Check sheet for the modelled part. Datum: model origin and axes. Units: mm. A direction names the side the tool comes from. Give positions to 0.01 mm unless a question says otherwise; leave off trailing zeros. Order: outer loops, then holes, each group sorted by start corner. A loop starts at its lowest first (then second) coordinate and runs counter-clockwise, first axis right, second up. Notation, with made-up numbers: (0, 64) - (29, 64) arc R16 ccw to (29, 79) - close; hole circle Ø11 at (25.5, 80.5). An arc over 180 degrees is marked (long way). Answer in a Markdown table with one row per item.
from build123d import *

# Parameters (mm, degrees)
BASE_DEPTH              = 0.8636
TIER1_DEPTH             = 0.3556
CHAMFER1_SIZE           = 0.3556
SKETCH3_R               = 1
BUTTON_DEPTH            = 0.3048
BUTTONC_R               = 0.0508
SKETCH4_W               = 5.08
SKETCH4_H               = 1.524
BOTTOM_CUT_DEPTH        = 0.0508
PINS_START              = -0.4445
SKETCH6_W               = 0.508
SKETCH6_H               = 0.1524
PINS_DEPTH              = 0.508
MIRROR2_START           = -0.4445
MIRROR2_COPY_1_SKETCH_W = 0.508
MIRROR2_COPY_1_SKETCH_H = 0.1524
MIRROR2_COPY_1_DEPTH    = 0.508


with BuildPart() as part:
    # Sketch1 → Base (new body)
    with BuildSketch(Plane.XY):
        Polygon((-1.3462, 2.54), (1.3462, 2.54), (2.54, 1.3462), (2.54, -1.3462), (1.3462, -2.54), (-1.3462, -2.54), (-2.54, -1.3462), (-2.54, 1.3462), align=None)
    extrude(amount=BASE_DEPTH)

    # Sketch2 → Tier1 (add)
    with BuildSketch(Plane.XY.offset(0.8636)):
        Polygon((-1.093695412, 1.9304), (-1.9304, 1.093695412), (-1.9304, -1.093695412), (-1.093695412, -1.9304), (1.093695412, -1.9304), (1.9304, -1.093695412), (1.9304, 1.093695412), (1.093695412, 1.9304), align=None)
    extrude(amount=TIER1_DEPTH)

    # Chamfer1
    chamfer1_edges = [part.edges().sort_by_distance(p)[0] for p in [
        (-1.512047706, 1.512047706, 1.2192),
        (0, 1.9304, 1.2192),
        (1.512047706, 1.512047706, 1.2192),
        (1.9304, 0, 1.2192),
        (1.512047706, -1.512047706, 1.2192),
        (0, -1.9304, 1.2192),
        (-1.512047706, -1.512047706, 1.2192),
        (-1.9304, 0, 1.2192),
    ]]
    chamfer(chamfer1_edges, length=CHAMFER1_SIZE - 0.0001)  # a hair under: the kernel refuses the full size

    # Sketch3 → Button (add)
    with BuildSketch(Plane.XY.offset(1.2192)):
        Circle(SKETCH3_R)
    extrude(amount=BUTTON_DEPTH)

    # ButtonC
    buttonc_edges = [part.edges().sort_by_distance(p)[0] for p in [
        (-1, 0, 1.524),
    ]]
    fillet(buttonc_edges, radius=BUTTONC_R)

    # Sketch4 → Bottom cut (cut)
    with BuildSketch(Plane(origin=(0, 0, 0), x_dir=(-1, 0, 0), z_dir=(0, 0, -1))):
        Rectangle(SKETCH4_W, SKETCH4_H)
    extrude(amount=-BOTTOM_CUT_DEPTH, mode=Mode.SUBTRACT)

    # Sketch6 → pins (add)
    with BuildSketch(Plane.XZ.offset(2.54).offset(PINS_START)):
        with Locations((-1.0922, 0.3048)):
            Rectangle(SKETCH6_W, SKETCH6_H)
        Polygon((-1.3462, 0.2286), (-1.3462, 0.381), (-2.2352, 0.381), (-2.2352, 0.3048), (-2.2352, 0.2286), align=None)
        with BuildLine():
            Line((-2.2352, 0.3048), (-2.2352, 0.381))
            add(Edge.make_bspline(
                [(-2.2352, 0.381), (-2.307735088, 0.381), (-2.477008689, 0.347316172), (-2.556176281, 0.222815828), (-2.591192004, 0.183226461), (-2.642048799, 0.15910292), (-2.712296659, 0.1524), (-2.742, 0.1524)],
                knots=[0, 0, 0, 0, 0.25, 0.5, 0.75, 0.875, 1, 1, 1, 1], degree=3))
            Line((-2.742, 0.1524), (-2.742, 0.0762))
            add(Edge.make_bspline(
                [(-2.2352, 0.3048), (-2.573866667, 0.3048), (-2.403333333, 0.0762), (-2.742, 0.0762)],
                knots=[0, 0, 0, 0, 1, 1, 1, 1], degree=3))
        make_face()
        with BuildLine():
            Line((-2.2352, 0.2286), (-2.2352, 0.3048))
            add(Edge.make_bspline(
                [(-2.2352, 0.3048), (-2.573866667, 0.3048), (-2.403333333, 0.0762), (-2.742, 0.0762)],
                knots=[0, 0, 0, 0, 1, 1, 1, 1], degree=3))
            Line((-2.742, 0.0762), (-2.742, 0))
            add(Edge.make_bspline(
                [(-2.2352, 0.2286), (-2.264903341, 0.2286), (-2.335151201, 0.22189708), (-2.386007996, 0.197773539), (-2.421023719, 0.158184172), (-2.500191311, 0.033683828), (-2.669464912, 0), (-2.742, 0)],
                knots=[0, 0, 0, 0, 0.125, 0.25, 0.5, 0.75, 1, 1, 1, 1], degree=3))
        make_face()
        with Locations((-2.996, 0.0762)):
            Rectangle(SKETCH6_W, SKETCH6_H)
    pins = extrude(amount=-PINS_DEPTH)

    # pins2: pins across plane
    add(pins.mirror(Plane.ZX))

    # Mirror2: pins across plane
    add(pins.mirror(Plane(origin=(0, 0, 0), x_dir=(0, 0, 1), z_dir=(1, 0, 0))))

    # Mirror2 copy 1 sketch → Mirror2 copy 1 (add)
    with BuildSketch(Plane(origin=(0, 2.54, 0), x_dir=(-1, 0, 0), z_dir=(0, 1, 0)).offset(MIRROR2_START)):
        with Locations((-1.0922, 0.3048)):
            Rectangle(MIRROR2_COPY_1_SKETCH_W, MIRROR2_COPY_1_SKETCH_H)
        Polygon((-1.3462, 0.2286), (-1.3462, 0.381), (-2.2352, 0.381), (-2.2352, 0.3048), (-2.2352, 0.2286), align=None)
        with BuildLine():
            Line((-2.2352, 0.3048), (-2.2352, 0.381))
            add(Edge.make_bspline(
                [(-2.2352, 0.381), (-2.307735088, 0.381), (-2.477008689, 0.347316172), (-2.556176281, 0.222815828), (-2.591192004, 0.183226461), (-2.642048799, 0.15910292), (-2.712296659, 0.1524), (-2.742, 0.1524)],
                knots=[0, 0, 0, 0, 0.25, 0.5, 0.75, 0.875, 1, 1, 1, 1], degree=3))
            Line((-2.742, 0.1524), (-2.742, 0.0762))
            add(Edge.make_bspline(
                [(-2.2352, 0.3048), (-2.573866667, 0.3048), (-2.403333333, 0.0762), (-2.742, 0.0762)],
                knots=[0, 0, 0, 0, 1, 1, 1, 1], degree=3))
        make_face()
        with BuildLine():
            Line((-2.2352, 0.2286), (-2.2352, 0.3048))
            add(Edge.make_bspline(
                [(-2.2352, 0.3048), (-2.573866667, 0.3048), (-2.403333333, 0.0762), (-2.742, 0.0762)],
                knots=[0, 0, 0, 0, 1, 1, 1, 1], degree=3))
            Line((-2.742, 0.0762), (-2.742, 0))
            add(Edge.make_bspline(
                [(-2.2352, 0.2286), (-2.264903341, 0.2286), (-2.335151201, 0.22189708), (-2.386007996, 0.197773539), (-2.421023719, 0.158184172), (-2.500191311, 0.033683828), (-2.669464912, 0), (-2.742, 0)],
                knots=[0, 0, 0, 0, 0.125, 0.25, 0.5, 0.75, 1, 1, 1, 1], degree=3))
        make_face()
        with Locations((-2.996, 0.0762)):
            Rectangle(MIRROR2_COPY_1_SKETCH_W, MIRROR2_COPY_1_SKETCH_H)
    extrude(amount=-MIRROR2_COPY_1_DEPTH)


solid = part.part
(1) Gauge pin test, flat ends, axial feed: P1, Ø0.5, axis at x = -2, y = 2, coming from the -Z side; P2, Ø0.7, axis at y = 0, z = 0.5, coming from the -X side; P3, Ø0.6, axis at x = -3, y = 2, coming from the +Z side; P4, Ø0.9, axis at y = 0, z = 0.5, coming from the +X side. Record the tip position at first contact, or that the pin passes through.
Geometry says:
| item | result |
|---|---|
| P1 | z = 0 |
| P2 | x = -2.54 |
| P3 | z = 0.15 |
| P4 | x = 2.54 |
(2) Thickness scan on L1, parallel to X at y = 1, z = 0.35; L2, parallel to Z at x = -0.25, y = 0.3; L3, parallel to X at y = 2, z = 0.1. Record the ranges inside material, lowest first.
Geometry says:
| item | result |
|---|---|
| L1 | -2.54 to 2.54 |
| L2 | 0.05 to 1.52 |
| L3 | -3.25 to -2.46, -1.89 to 1.89, 2.46 to 3.25 |
(3) Cross-section at C-C, the plane z = 0.7. Record the cut outline in (x, y).
Geometry says:
| item | result |
|---|---|
| outline | (-2.54, -1.35) - (-1.35, -2.54) - (1.35, -2.54) - (2.54, -1.35) - (2.54, 1.35) - (1.35, 2.54) - (-1.35, 2.54) - (-2.54, 1.35) - close |
(4) Mould release check, pull along Y, two halves, no side actions. Record for faces 1 (the flat face through (-2.54, 0, 0.4)), 2 (the flat face through (1.379, -1.39, 1.044)), 3 (the flat face through (0, -2, 0)): pulls with the +Y half, pulls with the -Y half, needs draft (parallel to the pull), parting line crosses it, or undercut.
Geometry says:
| item | result |
|---|---|
| face 1 | undercut |
| face 2 | pulls with the -Y half |
| face 3 | needs draft |
(5) Access from +Z, -Z, +X, -X, +Y, -Y to the whole of each face (thin tool, end or side, straight path). Record for faces 4 (the flat face through (0, 0, 0.051)), 5 (the flat face through (1.39, 1.379, 1.044)), 6 (the flat face through (2.1, 0, 0.864)), 7 (the flat face through (2.54, 0, 0.4)), 8 (the flat face through (0, 0, 1.524)).
Geometry says:
| item | result |
|---|---|
| face 4 | -Z, +X, -X |
| face 5 | +Z, +X, +Y |
| face 6 | +Z |
| face 7 | +Z, -Z, +X |
| face 8 | +Z, +X, -X, +Y, -Y |
